from build123d import *

# Parameters (mm, degrees)
BOSS_EXTRUDE1_DEPTH = 10
SKETCH2_W           = 12
SKETCH2_H           = 10
BOSS_EXTRUDE2_DEPTH = 3
SKETCH3_R           = 3
CUT_EXTRUDE1_DEPTH  = 12
SKETCH4_R           = 0.5
BOSS_EXTRUDE3_DEPTH = 10
FILLET6_R           = 0.5


with BuildPart() as part:
    # Sketch1 → Boss-Extrude1 (new body)
    with BuildSketch(Plane(origin=(0, 0, 0), x_dir=(0, 0, -1), z_dir=(1, 0, 0))):
        with BuildLine():
            Line((-4.5, -43.179278244), (4.5, -43.179278244))
            Line((4.5, -43.179278244), (4.5, -38.179278244))
            ThreePointArc((4.5, -38.179278244), (0, -33.679278244), (-4.5, -38.179278244))
            Line((-4.5, -38.179278244), (-4.5, -43.179278244))
        make_face()
    extrude(amount=BOSS_EXTRUDE1_DEPTH)

    # Sketch2 → Boss-Extrude2 (add)
    with BuildSketch(Plane.ZY):
        with Locations((0, -38.179278244)):
            Rectangle(SKETCH2_W, SKETCH2_H)
    extrude(amount=BOSS_EXTRUDE2_DEPTH)

    # Sketch3 → Cut-Extrude1 (cut)
    with BuildSketch(Plane.ZY.offset(3)):
        with Locations((0, -38.179278244)):
            Circle(SKETCH3_R)
    extrude(amount=-CUT_EXTRUDE1_DEPTH, mode=Mode.SUBTRACT)

    # Sketch4 → Boss-Extrude3 (add)
    with BuildSketch(Plane.ZY.offset(-9)):
        with Locations((0, -38.179278244)):
            Circle(SKETCH4_R)
    extrude(amount=BOSS_EXTRUDE3_DEPTH)

    # Fillet6
    fillet6_edges = [part.edges().sort_by_distance(p)[0] for p in [
        (-1, -38.179278244, -0.5),
    ]]
    fillet(fillet6_edges, radius=FILLET6_R)


solid = part.part
Read the model definition and answer for the solid it produces. Units are mm, in the model's axes. A direction names the side the tool comes from. Round coordinates to 2 decimals unless told otherwise and drop trailing zeros. Order: outer loops, then holes, each group sorted by start corner. A loop starts at its lowest first (then second) coordinate and runs counter-clockwise, first axis right, second up.
1) The part is cut by section B-B on z = 0. Write down the section's boundary in (x, y).
2) The mould has two halves that part along Y. Classify faces 5 (the face through (2.916, -35.205, -0.391)), 6 (the face through (4.316, -37.684, -0.065)), 7 (the face through (4, -43.179, 0)), 8 (the face through (5, -41, -4.5)): released by +Y, released by -Y, zero draft, split by the parting line, or undercut.
3) The part is cut by section D-D on z = -2. Write down the section's boundary in (x, y), plus the area to 3 significant figures.
4) The part is cut by section A-A on x = 2.5. Write down the section's boundary in (y, z).
5) For faces 1 (the face through (-1, -38, -6)), 2 (the face through (4.93, -33.68, -0.1)), 3 (the face through (9, -38, 1)), 4 (the face through (5, -41, 4.5)), determine the directions among +Z, -Z, +X, -X, +Y, -Y from which every point of the face is accessible in a straight line to the end or side of a thin tool.
6) The part is cut by section C-C on y = -40.5. Write down the section's boundary in (x, z).
7) Flat-ended cylindrical pins translate along their axes: pin 1 (6 mm diameter, centred on x = 8, y = -39.5, fed in from -Z); pin 2 (5 mm diameter, centred on x = 8.5, y = -36.5, fed in from +Z). Find the tip coordinate at first contact, or state that the pin passes through.
8) Straight lines are drawn through the part: L1, parallel to Y at x = 4.75, z = 0; L2, parallel to Z at x = 3, y = -42; L3, parallel to Y at x = 2.75, z = -1. For each, find the intervals that lie inside material, in ascending order.
Resolved:
1. outline: (-3, -43.18) - (10, -43.18) - (10, -33.68) - (0, -33.68) - (0, -33.18) - (-3, -33.18) - (-3, -35.18) - (9, -35.18) - (9, -37.68) - (-0.5, -37.68) arc R0.5 ccw to (-0.5, -38.68) - (9, -38.68) - (9, -41.18) - (-3, -41.18) - close
2. face 5: undercut
2. face 6: undercut
2. face 7: released by -Y
2. face 8: zero draft
3. outline: (-3, -43.18) - (10, -43.18) - (10, -34.15) - (0, -34.15) - (0, -33.18) - (-3, -33.18) - (-3, -35.94) - (9, -35.94) - (9, -40.42) - (-3, -40.42) - close
3. area: 66.6 mm2
4. outline: (-43.18, -4.5) - (-38.18, -4.5) arc R4.5 ccw to (-38.18, 4.5) - (-43.18, 4.5) - close; circle Ø1 at (-38.18, 0); hole circle Ø6 at (-38.18, 0)
5. face 1: -Z, +X, -X, +Y, -Y
5. face 2: +X, +Y
5. face 3: -X
5. face 4: +Z, +X, +Y, -Y
6. outline: (-3, -6) - (0, -6) - (0, -4.5) - (10, -4.5) - (10, 4.5) - (0, 4.5) - (0, 6) - (-3, 6) - (-3, 1.9) - (9, 1.9) - (9, -1.9) - (-3, -1.9) - close
7. pin 1: stops at z = -4.5
7. pin 2: stops at z = 4.5
8. L1: y = -43.18 to -41.18, -38.68 to -37.68, -35.18 to -33.68
8. L2: z = -4.5 to 4.5
8. L3: y = -43.18 to -41.01, -35.35 to -33.79
